Here's the drawing with two shaded views (mm, measured from the low corner). I have some questions. Give positions to 0.01 mm unless a question says otherwise; leave off trailing zeros. Loops run counter-clockwise (first coordinate to the right, second up) from the corner with the lowest first, then second, coordinate; pieces in that order, holes last. Notation, with made-up numbers: (45, 54.5) -> (92, 54.5) arc R11 cw to (92, 63.5) -> close; hole circle Ø2 at (67, -10). An arc over 180 degrees is marked (long way). Put each result on its own line as item: value.
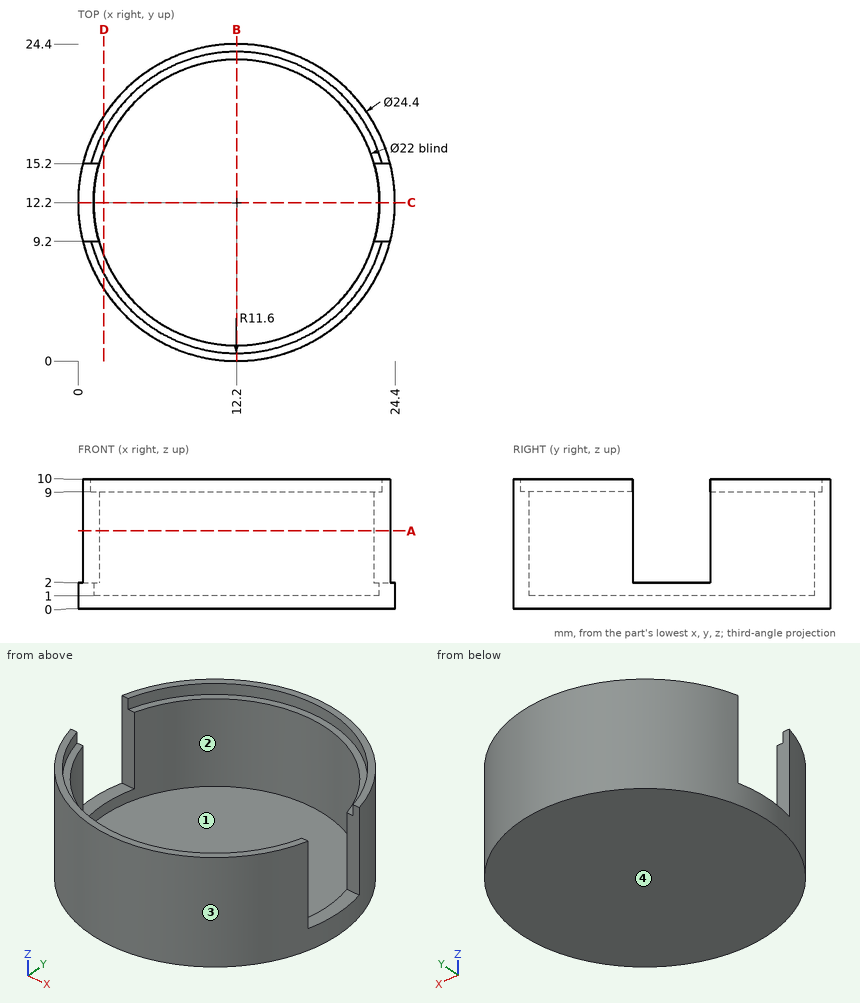
1. I'm going to push flat-ended pins straight in: pin 1 (0.8 mm diameter, centred on x = 1, y = 13.5, fed in from +Z); pin 2 (2 mm diameter, centred on y = 21.5, z = 4.5, fed in from +X); pin 3 (1.4 mm diameter, centred on x = 23, z = 4.5, fed in from -Y); pin 4 (1 mm diameter, centred on x = 20.5, y = 8.5, fed in from -Z). Where does each tip first touch, or does it pass through?
Recorded:
pin 1: stops at z = 2
pin 2: stops at x = 21.14
pin 3: stops at y = 5.36
pin 4: stops at z = 0
2. Thinking about a two-plate mould opening in Y: for the marked faces 1, 2, 3 and 4, which applies, pulls with the +Y half, pulls with the -Y half, needs draft (parallel to the pull), parting line crosses it, or undercut?
Recorded:
face 1: undercut
face 2: undercut
face 3: parting line crosses it
face 4: needs draft
3. If we section it at A-A (z = 6): List the corners of the cut face in (x, y) for me.
Recorded:
outline: (0.37, 9.2) arc R12.2 ccw to (24.03, 9.2) -> (22.78, 9.2) arc R11 cw to (1.62, 9.2) -> close; (0.37, 15.2) -> (1.62, 15.2) arc R11 cw to (22.78, 15.2) -> (24.03, 15.2) arc R12.2 ccw to start
4. If we section it at C-C (y = 12.2): List the corners of the cut face in (x, z) for me.
Recorded:
outline: (0, 0) -> (24.4, 0) -> (24.4, 2) -> (23.2, 2) -> (23.2, 1) -> (1.2, 1) -> (1.2, 2) -> (0, 2) -> close
5. If we section it at D-D (x = 2): List the corners of the cut face in (y, z) for me.
Recorded:
outline: (5.51, 0) -> (18.89, 0) -> (18.89, 10) -> (17.72, 10) -> (17.72, 9) -> (16.32, 9) -> (16.32, 1) -> (8.08, 1) -> (8.08, 9) -> (6.68, 9) -> (6.68, 10) -> (5.51, 10) -> close
6. I need wall thicknesses on line 1 (Y direction, x = 12.2, z = 5.5); line 2 (Z direction, x = 3, y = 14.5); line 3 (Y direction, x = 14, z = 5). Which ranges of each line are inside material? Lowest first, please.
Recorded:
line 1: y = 0 to 1.2, 23.2 to 24.4
line 2: z = 0 to 1
line 3: y = 0.13 to 1.35, 23.05 to 24.27
7. If we section it at B-B (x = 12.2): List the corners of the cut face in (y, z) for me, then the cut area to 3 significant figures.
Recorded:
outline: (0, 0) -> (24.4, 0) -> (24.4, 10) -> (23.8, 10) -> (23.8, 9) -> (23.2, 9) -> (23.2, 1) -> (1.2, 1) -> (1.2, 9) -> (0.6, 9) -> (0.6, 10) -> (0, 10) -> close
area: 44.8 mm^2
